CAD build for the part. Positions are in the model's coordinates, mm. Face numbers are marked on the shaded views. Give positions to 0.01 mm unless a question says otherwise; leave off trailing zeros. Loops run counter-clockwise (first coordinate to the right, second up) from the corner with the lowest first, then second, coordinate; pieces in that order, holes last.
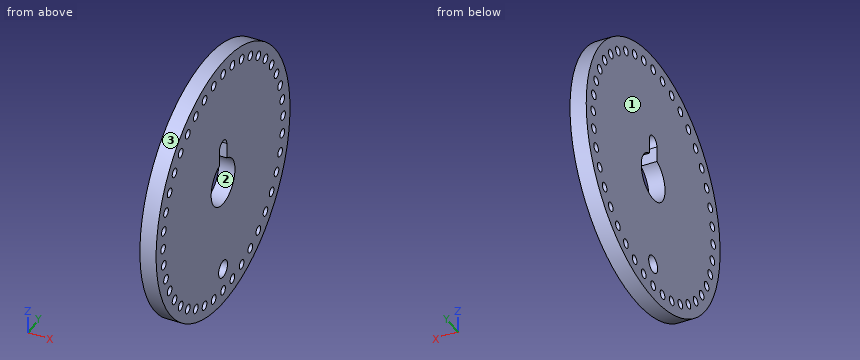
Autodesk Inventor part; units mm, degrees
ref_plane "YZ Plane" through (0, 0, 0) normal (1, 0, 0) x (0, 1, 0)
ref_plane "XZ Plane" through (0, 0, 0) normal (0, 1, 0) x (-1, 0, 0)
ref_plane "XY Plane" through (0, 0, 0) normal (0, 0, 1) x (1, 0, 0)
sketch "Sketch2" plane through (0, 0, 0) normal (1, 0, 0) x (0, 1, 0)
  circle A0 centre (0, 0) radius 45
  dimension "d7" = 90
extrude "Extrusion1" add sketch "Sketch2" along normal blind 5.588
sketch "Sketch3" plane through (5.588, 0, 0) normal (1, 0, 0) x (0, 0, -1)
  circle A0 centre (0, 0) radius 45
  line L0 (0, 0) -> (-45, 0)
  circle A1 centre (0, 0) radius 45
  point P0 (-40.325, 0)
  dimension "d10" = 40.325
hole "Hole1" at (5.588, 0, 40.325) direction (-1, 0, 0) diameter 3.1 end through all
pattern_circular "Circular Pattern1" count 40 over 360 about axis through (-10, 0, 0) along (1, 0, 0) of "Hole1"
sketch "Sketch4" plane through (5.588, 0, 0) normal (1, 0, 0) x (0, 0, -1)
  point P0 (0, 0)
  point P1 (0, 0)
hole "Hole2" at (5.588, 0, 0) direction (-1, 0, 0) diameter 16 end through all
sketch "Sketch5" plane through (5.588, 0, 0) normal (1, 0, 0) x (0, 0, -1)
  line L0 (0, -2.5) -> (-13, -2.5)
  line L1 (-13, -2.5) -> (-13, 2.5)
  line L2 (-13, 2.5) -> (0, 2.5)
  line L3 (0, 2.5) -> (0, -2.5)
  arc A0 (-13, 2.5) -> (-13, -2.5) centre (-13, 0) ccw
  point P0 (0, 0)
  point P1 (0, 0)
  dimension "d28" = 5
  dimension "d29" = 13
extrude "Extrusion2" cut sketch "Sketch5" against normal through all
sketch "Sketch6" plane through (5.588, 0, 0) normal (1, 0, 0) x (0, 0, -1)
  line L0 (-13, 2.5) -> (-7.5993, 2.5)
  arc A0 (-7.5993, -2.5) -> (-7.5993, 2.5) centre (0, 0) ccw
  line L1 (-7.5993, -2.5) -> (-13, -2.5)
  arc A1 (-13, 2.5) -> (-13, -2.5) centre (-13, 0) ccw
  circle A2 centre (-39.8285, 6.3082) radius 1.55
  circle A3 centre (-38.3514, 12.4611) radius 1.55
  circle A4 centre (-35.9298, 18.3072) radius 1.55
  circle A5 centre (-32.6236, 23.7024) radius 1.55
  circle A6 centre (-28.5141, 28.5141) radius 1.55
  circle A7 centre (-23.7024, 32.6236) radius 1.55
  circle A8 centre (-18.3072, 35.9298) radius 1.55
  circle A9 centre (-12.4611, 38.3514) radius 1.55
  circle A10 centre (-6.3082, 39.8285) radius 1.55
  circle A11 centre (0, 40.325) radius 1.55
  circle A12 centre (6.3082, 39.8285) radius 1.55
  circle A13 centre (12.4611, 38.3514) radius 1.55
  circle A14 centre (18.3072, 35.9298) radius 1.55
  circle A15 centre (23.7024, 32.6236) radius 1.55
  circle A16 centre (28.5141, 28.5141) radius 1.55
  circle A17 centre (32.6236, 23.7024) radius 1.55
  circle A18 centre (35.9298, 18.3072) radius 1.55
  circle A19 centre (38.3514, 12.4611) radius 1.55
  circle A20 centre (39.8285, 6.3082) radius 1.55
  circle A21 centre (40.325, 0) radius 1.55
  circle A22 centre (39.8285, -6.3082) radius 1.55
  circle A23 centre (38.3514, -12.4611) radius 1.55
  circle A24 centre (35.9298, -18.3072) radius 1.55
  circle A25 centre (32.6236, -23.7024) radius 1.55
  circle A26 centre (28.5141, -28.5141) radius 1.55
  circle A27 centre (23.7024, -32.6236) radius 1.55
  circle A28 centre (18.3072, -35.9298) radius 1.55
  circle A29 centre (12.4611, -38.3514) radius 1.55
  circle A30 centre (6.3082, -39.8285) radius 1.55
  circle A31 centre (0, -40.325) radius 1.55
  circle A32 centre (-6.3082, -39.8285) radius 1.55
  circle A33 centre (-12.4611, -38.3514) radius 1.55
  circle A34 centre (-18.3072, -35.9298) radius 1.55
  circle A35 centre (-23.7024, -32.6236) radius 1.55
  circle A36 centre (-28.5141, -28.5141) radius 1.55
  circle A37 centre (-32.6236, -23.7024) radius 1.55
  circle A38 centre (-35.9298, -18.3072) radius 1.55
  circle A39 centre (-38.3514, -12.4611) radius 1.55
  circle A40 centre (-39.8285, -6.3082) radius 1.55
  circle A41 centre (-40.325, 0) radius 1.55
  circle A42 centre (0, 0) radius 45
  point P0 (32.325, 0)
  dimension "d32" = 8
  dimension "d33" = 0
hole "Hole3" at (5.588, 0, -32.325) direction (-1, 0, 0) diameter 6 end through all
equation "\"d7\" = spoolDiameter"
equation "\"d8\" = spoolThickness"
equation "\"d34\" = magnetDiameter"
equation "\"materialThickness\" = 3.175"
equation "\"laserKerf\" = 0.12"
equation "\"cardPinDiameter\" = 3"
equation "\"spoolDiameter\" = 90"
equation "\"centeralShaftDiameter\" = 8"
equation "\"cardHeight\" = 53.98"
equation "\"cardWidth\" = 85.6"
equation "\"cardThickness\" = 0.76"
equation "\"cardFillet\" = 2.88"
equation "\"cardClearence\" = 0.5"
equation "\"bearingOd\" = 22"
equation "\"bearingWidth\" = 8"
equation "\"axleHeight\" = 95"
equation "\"nutTrapDepth\" = 2.5"
equation "\"nutTrapwidth\" = 5.5"
equation "\"nutTrapClearence\" = 2"
equation "\"magnetLength\" = 3"
equation "\"magnetDiameter\" = 6"
equation "\"magnetProtusion\" = 0.25"
equation "\"spoolThickness\" = 5.588"
properties part number "spoolBase" material "Polycarbonate, Clear"
1. Probe line 1 along Z through (x, y) = (3.3, -18.5); line 2 along Z through (x, y) = (0.5, -28.5); line 3 along Y through (x, z) = (4.45, -38.5). List the from-to ranges inside material, lowest first.
Responses:
line 1: z = -41.02 to -37.47, -34.39 to 34.39, 37.47 to 41.02
line 2: z = -34.82 to -30.06, -26.96 to 26.96, 30.06 to 34.82
line 3: y = -23.3 to -14, -10.92 to -7.11, -5.51 to 5.51, 7.11 to 10.92, 14 to 23.3
2. Pull direction Z, two halves, no side cores. Call the marked faces 1, 2 and 3: released by +Z, released by -Z, zero draft, split by the parting line, or undercut.
Responses:
face 1: zero draft
face 2: undercut
face 3: split by the parting line
3. Drop flat-ended pins along their axis: pin 1 (3.5 mm diameter, centred on y = 39.83, z = 6.31, fed in from -X); pin 2 (3 mm diameter, centred on y = -18.31, z = 35.93, fed in from -X); pin 3 (1.5 mm diameter, centred on x = 1.5, z = 14, fed in from -Y); pin 4 (1 mm diameter, centred on x = 2, y = -32.5, fed in from -Z). Give the stop position or say it passes through.
Responses:
pin 1: stops at x = 0
pin 2: passes through
pin 3: stops at y = -43.01
pin 4: stops at z = -31.64
4. Saw through at A-A, the plane z = 0. List the corners of the cut face in (x, y) (3 decimals), and give its area (3 significant figures).
Responses:
outline: (0, -45) - (5.588, -45) - (5.588, -41.875) - (0, -41.875) - close; (0, -38.775) - (5.588, -38.775) - (5.588, -8) - (0, -8) - close; (0, 8) - (5.588, 8) - (5.588, 38.775) - (0, 38.775) - close; (0, 41.875) - (5.588, 41.875) - (5.588, 45) - (0, 45) - close
area: 379 mm2
5. Saw through at B-B, the plane y = 0. List the corners of the cut face in (x, z) (3 decimals).
Responses:
outline: (0, -45) - (5.588, -45) - (5.588, -41.875) - (0, -41.875) - close; (0, -38.775) - (5.588, -38.775) - (5.588, -35.325) - (0, -35.325) - close; (0, -29.325) - (5.588, -29.325) - (5.588, -8) - (0, -8) - close; (0, 15.5) - (5.588, 15.5) - (5.588, 38.775) - (0, 38.775) - close; (0, 41.875) - (5.588, 41.875) - (5.588, 45) - (0, 45) - close
